Check sheet for the drawn part. Datum: minimum x, y, z corner. Units: mm. A direction names the side the tool comes from. Give positions to 0.01 mm unless a question says otherwise; leave off trailing zeros. Write each loop counter-clockwise with the first axis right and the second up, starting at its lowest first coordinate (ties: lowest second). Pieces come first, ordered by that corner, then holes. Notation, with made-up numbers: (-20, -38.75) -> (13, -38.75) arc R10 cw to (13, -34.75) -> close; hole circle Ø8 at (31.5, 75.5). An arc over 180 degrees is marked (long way). Answer as CSV lines item,"result". Start each with the question number.
1) Sectioned sample at A-A on x = 4. Record the cut outline in (y, z), and give its area (3 significant figures).
2) Sectioned sample at B-B on y = 4. Record the cut outline in (x, z), and give its area (3 significant figures).
3) Tool access check on the marked faces 5, 6 and 7. Record the directions out of +Z, -Z, +X, -X, +Y, -Y that give a thin tool (end or side, any length) a straight path to the whole face; none if there is none.
4) Sectioned sample at D-D on y = 1.75. Record the cut outline in (x, z), and give its area (3 significant figures).
5) Mould release check, pull along Y, two halves, no side actions. Record for the marked faces 1, 2, 3 and 4: released by +Y, released by -Y, zero draft, split by the parting line, or undercut.
6) Sectioned sample at C-C on z = 4.5. Record the cut outline in (x, y).
7) Gauge pin test, flat ends, axial feed: pin 1 Ø3 at (y, z) = (1, 3) entering from -X; pin 2 Ø1.8 at (x, y) = (4, 4) entering from +Z; pin 3 Ø3 at (y, z) = (7, 8.5) entering from +X. Record the tip position at first contact, or that the pin passes through.
8) Material ranges on L1, parallel to Z at x = 4, y = 1.45; L2, parallel to Y at x = 3, z = 1; L3, parallel to Z at x = 7, y = 4.25, recorded low to high.
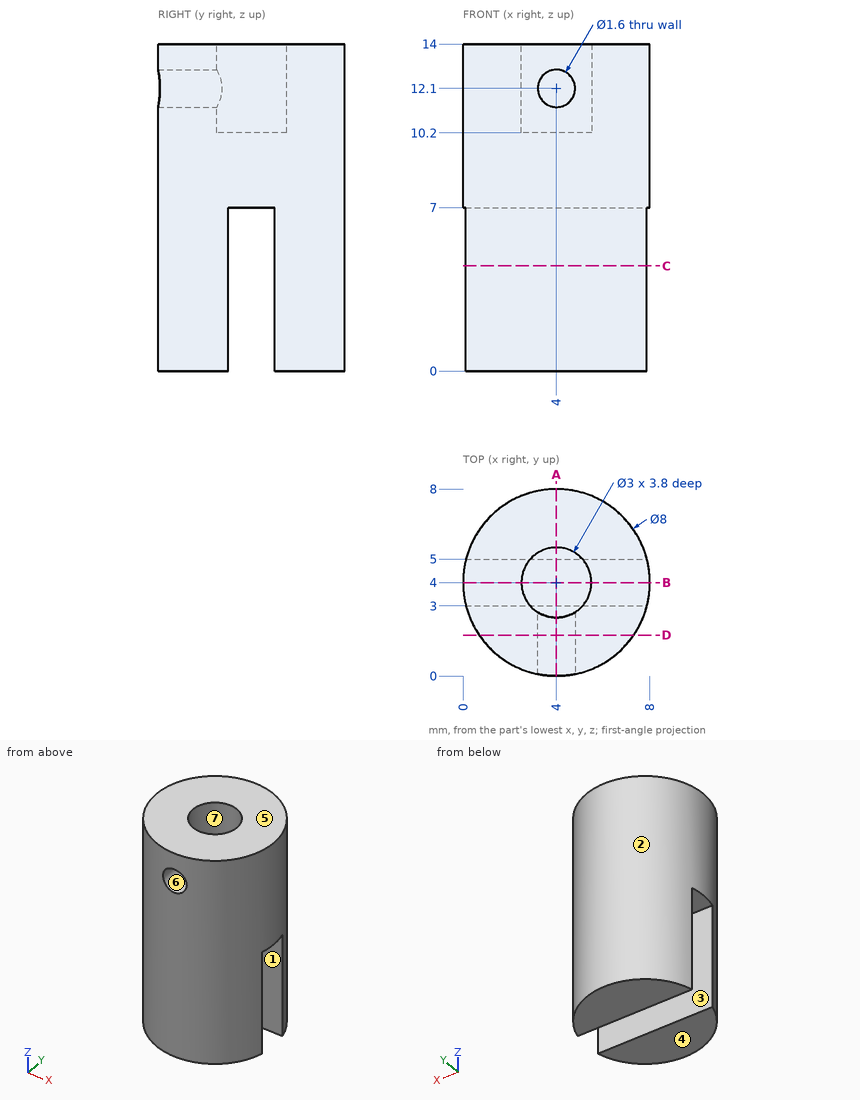
Ans:
1,outline,"(0, 0) -> (3, 0) -> (3, 7) -> (5, 7) -> (5, 0) -> (8, 0) -> (8, 14) -> (5.5, 14) -> (5.5, 10.2) -> (2.5, 10.2) -> (2.5, 11.3) -> (0, 11.3) -> close; (0, 12.9) -> (2.5, 12.9) -> (2.5, 14) -> (0, 14) -> close"
1,area,"82.6 mm²"
2,outline,"(0, 7) -> (8, 7) -> (8, 14) -> (5.5, 14) -> (5.5, 10.2) -> (2.5, 10.2) -> (2.5, 14) -> (0, 14) -> close"
2,area,"44.6 mm²"
3,face 5,"+Z, +X, -X, +Y, -Y"
3,face 6,"-Y"
3,face 7,"+Z"
4,outline,"(0.69, 0) -> (7.31, 0) -> (7.31, 14) -> (0.69, 14) -> close; hole circle Ø1.6 at (4, 12.1)"
4,area,"90.6 mm²"
5,face 1,"undercut"
5,face 2,"split by the parting line"
5,face 3,"undercut"
5,face 4,"zero draft"
6,outline,"(0.13, 3) arc R4 ccw to (7.87, 3) -> close; (0.13, 5) -> (7.87, 5) arc R4 ccw to start"
7,pin 1,"stops at x = 0.29"
7,pin 2,"stops at z = 10.2"
7,pin 3,"stops at x = 7.71"
8,L1,"z = 0 to 11.3, 12.9 to 14"
8,L2,"y = 0.13 to 3, 5 to 7.87"
8,L3,"z = 7 to 14"
